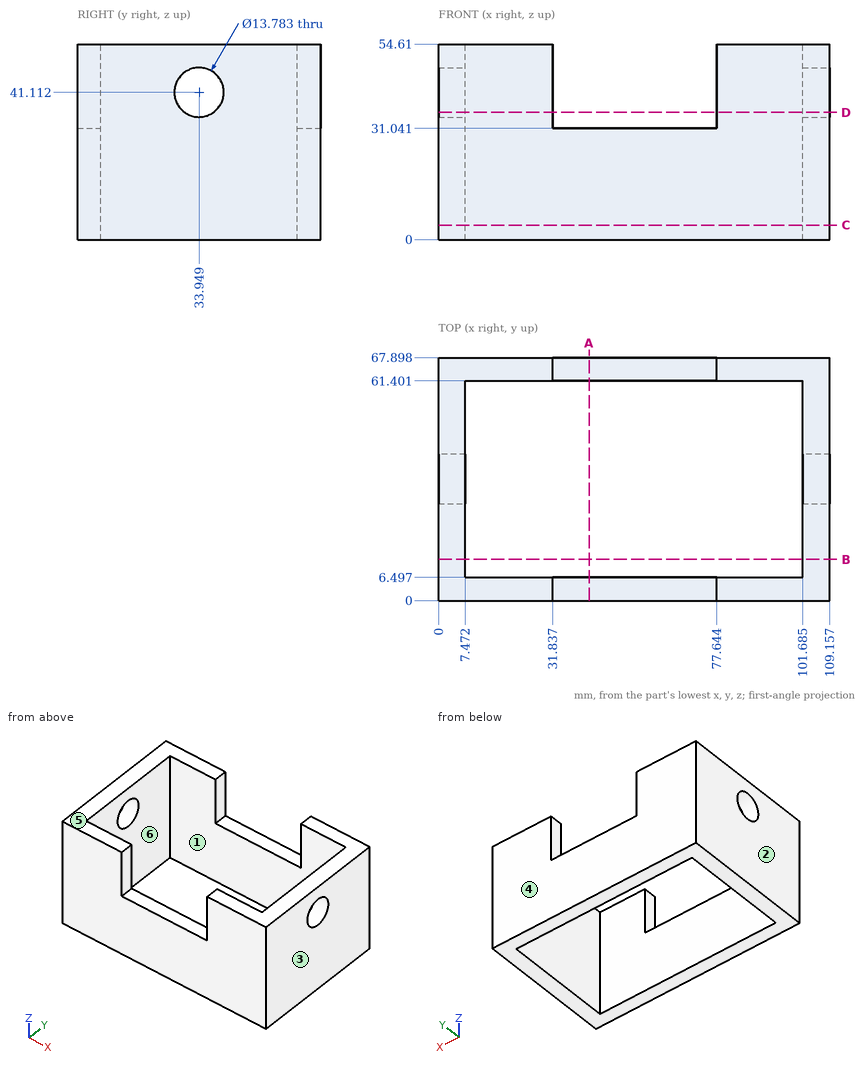
The drawing under review shows one solid part. Ordinate dimensions are in mm from its lowest x, y, z. A direction names the side the tool comes from. Coordinates: 2 decimals unless noted, no trailing zeros. Order: outer loops, then holes, each group sorted by start corner. A loop starts at its lowest first (then second) coordinate and runs counter-clockwise, first axis right, second up. Notation, with made-up numbers: (-5.5, 33.5) - (52.5, 33.5) arc R19 ccw to (52.5, 70.5) - close; hole circle Ø11 at (-24.75, 29). An arc over 180 degrees is marked (long way). Put each result on its own line as item: value.
1) Insertion check: P1, Ø7, axis at x = 54, y = 65, coming from the +Z side. The pin has a flat end and moves straight along its axis. Give the tip position at first contact, or say it passes through.
Response values:
P1: stops at z = 31.04
2) Take a section at A-A, the plane x = 42. Give the boundary of the cut face in (y, z).
Response values:
outline: (0, 0) - (6.5, 0) - (6.5, 31.04) - (0, 31.04) - close; (61.4, 0) - (67.9, 0) - (67.9, 31.04) - (61.4, 31.04) - close
3) Take a section at B-B, the plane y = 11.5. Give the boundary of the cut face in (x, z) (1 decimal).
Response values:
outline: (0, 0) - (7.5, 0) - (7.5, 54.6) - (0, 54.6) - close; (101.7, 0) - (109.2, 0) - (109.2, 54.6) - (101.7, 54.6) - close
4) Tool access review of the marked faces 5 and 6: name each direction out of +Z, -Z, +X, -X, +Y, -Y from which nothing blocks a thin tool from reaching the whole face with its end or side.
Response values:
face 5: +Z, +X, -X, +Y, -Y
face 6: +Z, -Z
5) Take a section at D-D, the plane z = 35.5. Count the separate pieces of the cut face and the enclosed holes in it, and give its area (3 significant figures).
Response values:
separate pieces: 4
enclosed holes: 0
area: 1,520 mm²
6) Take a section at C-C, the plane z = 4. Give the boundary of the cut face in (x, y) (1 decimal).
Response values:
outline: (0, 0) - (109.2, 0) - (109.2, 67.9) - (0, 67.9) - close; hole (7.5, 6.5) - (101.7, 6.5) - (101.7, 61.4) - (7.5, 61.4) - close
7) Wall thickness on L1, parallel to X at y = 59, z = 22 (1 decimal); L2, parallel to Y at x = 27, z = 49; L3, parallel to X at y = 3.5, z = 34 (1 decimal): over which ranges is each line inside the solid? List them lowest first. Write a range as from..to.
Response values:
L1: x = 0..7.5, 101.7..109.2
L2: y = 0..6.5, 61.4..67.9
L3: x = 0..31.8, 77.6..109.2
8) The part is to be moulded in two halves that separate along X. For the marked faces 1, 2, 3 and 4, say which applies: released by +X, released by -X, zero draft, split by the parting line, or undercut.
Response values:
face 1: undercut
face 2: released by -X
face 3: released by +X
face 4: zero draft
